from build123d import *

# Parameters (mm, degrees)
SKETCH_2_R               = 4
SKETCH_2_R_2             = 2
SKETCH_2_R_3             = 2.5
SKETCH_2_R_4             = 1.5
SKETCH_2_R_5             = 2.125
SKETCH_2_R_6             = 1
EXTRUDE_1_DEPTH          = 17.125
CUT_EXTRUDE_1_DEPTH      = 137.144257132
CUT_EXTRUDE_1_DEPTH_BACK = 137.144257132
SKETCH_3_W               = 6.985996156
SKETCH_3_H               = 14.275
CUT_EXTRUDE_START        = -128.325
CUT_EXTRUDE_2_OUTLINE_W  = 32
CUT_EXTRUDE_2_OUTLINE_H  = 0.125
CUT_EXTRUDE_2_DEPTH      = 16.325


# Read off the part's stored shape, not the designer's step: 切除-拉伸2
with BuildPart() as part:
    # 草图2 → 凸台-拉伸1 (new body)
    # profile 1 of 4: a face of its own
    with BuildSketch(Plane.XY.offset(8.375)):
        with BuildLine():
            Line((-15.5, -121), (-15.5, -116))
            Line((-15.5, -116), (-17.125, -116))
            ThreePointArc((-17.125, -116), (-23.953427125, -118.828427125), (-21.125, -112))
            Line((-21.125, -112), (-35.875, -112))
            ThreePointArc((-35.875, -112), (-34.107233047, -112.732233047), (-33.375, -114.5))
            ThreePointArc((-33.375, -114.5), (-35.875, -117), (-38.375, -114.5))
            Line((-38.375, -114.5), (-38.375, -118.75))
            Line((-38.375, -118.75), (-43.26696162, -120.643234405))
            ThreePointArc((-43.26696162, -120.643234405), (-41.298785706, -120.872085507), (-40.375, -122.625))
            ThreePointArc((-40.375, -122.625), (-41.477365663, -124.487751731), (-43.640735541, -124.417860124))
            Line((-43.640735541, -124.417860124), (-37.5, -128.325))
            Line((-37.5, -128.325), (-23, -128.325))
            Line((-23, -128.325), (-15.5, -121))
        make_face()
    # profile 2 of 4: a face of its own
    with BuildSketch(Plane.XY.offset(8.375)):
        with Locations((-21.125, -116)):
            Circle(SKETCH_2_R)
        with Locations((-21.125, -116)):
            Circle(SKETCH_2_R_2, mode=Mode.SUBTRACT)
    # profile 3 of 4: a face of its own
    with BuildSketch(Plane.XY.offset(8.375)):
        with Locations((-35.875, -114.5)):
            Circle(SKETCH_2_R_3)
        with Locations((-35.875, -114.5)):
            Circle(SKETCH_2_R_4, mode=Mode.SUBTRACT)
    # profile 4 of 4: a face of its own
    with BuildSketch(Plane.XY.offset(8.375)):
        with Locations((-42.5, -122.625)):
            Circle(SKETCH_2_R_5)
        with Locations((-42.5, -122.625)):
            Circle(SKETCH_2_R_6, mode=Mode.SUBTRACT)
    extrude(amount=-EXTRUDE_1_DEPTH)

    # 草图3 → 切除-拉伸1 (cut, two sides: drawn at the far end of the back side and taken through both)
    with BuildSketch(Plane(origin=(0, 0, 0), x_dir=(1, 0, 0), z_dir=(0, 1, 0)).offset(-CUT_EXTRUDE_1_DEPTH_BACK)):
        with Locations((-42.942998078, 0.1875)):
            Rectangle(SKETCH_3_W, SKETCH_3_H)
    extrude(amount=CUT_EXTRUDE_1_DEPTH + CUT_EXTRUDE_1_DEPTH_BACK, mode=Mode.SUBTRACT)

    # 切除-拉伸2 outline → 切除-拉伸2 (cut)
    with BuildSketch(Plane(origin=(0, 0, 0), x_dir=(1, 0, 0), z_dir=(0, 1, 0)).offset(CUT_EXTRUDE_START)):
        with Locations((-30, -8.3125)):
            Rectangle(CUT_EXTRUDE_2_OUTLINE_W, CUT_EXTRUDE_2_OUTLINE_H)
        with Locations((-30, 8.6875)):
            Rectangle(CUT_EXTRUDE_2_OUTLINE_W, CUT_EXTRUDE_2_OUTLINE_H)
    extrude(amount=CUT_EXTRUDE_2_DEPTH, mode=Mode.SUBTRACT)


solid = part.part
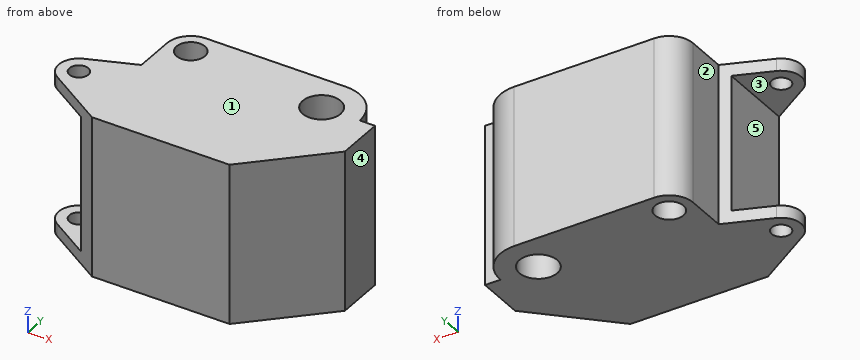
For this review, take the finished solid that the model builds, in its own axes (mm). Face numbers are marked on the shaded views. A direction names the side the tool comes from. Round coordinates to 2 decimals unless told otherwise and drop trailing zeros. Loops run counter-clockwise (first coordinate to the right, second up) from the corner with the lowest first, then second, coordinate; pieces in that order, holes last. Notation, with made-up numbers: (-28.5, 58.25) - (-24.5, 58.25) arc R13 ccw to (-24.5, 70.25) - close; hole circle Ø10 at (68, -36.5). An arc over 180 degrees is marked (long way). Answer as CSV lines item,"result".
(1) Insertion check: P1, Ø1, axis at x = -19.5, z = -0.5, coming from the +Y side; P2, Ø0.5, axis at x = -16.5, z = -0.5, coming from the +Y side; P3, Ø4, axis at y = -121.5, z = -1, coming from the -X side. Each pin has a flat end and moves straight along its axis. Give the tip position at first contact, or say it passes through.
Checked values:
P1,"stops at y = -112.16"
P2,"stops at y = -116"
P3,"stops at x = -39.45"
(2) Wall thickness on line 1 (Z direction, x = -41.25, y = -120.5) (3 decimals); line 2 (X direction, y = -114.5, z = -5) (3 decimals); line 3 (Y direction, x = -42.75, z = 7.5): over which ranges is each line inside the solid? List them lowest first.
Checked values:
line 1,"z = -8.625 to -7.325, 6.95 to 8.25"
line 2,"x = -38.375 to -37.375, -34.375 to -22.448, -19.802 to -17.417"
line 3,"y = -124.98 to -123.59, -121.66 to -120.44"
(3) Consider section B-B on x = -40. Give the boundary of the cut face in (y, z) (3 decimals).
Checked values:
outline,"(-126.734, -8.625) - (-119.379, -8.625) - (-119.379, -7.325) - (-126.734, -7.325) - close; (-126.734, 6.95) - (-119.379, 6.95) - (-119.379, 8.25) - (-126.734, 8.25) - close"
(4) Tool access review of the marked faces 4 and 5: name each direction out of +Z, -Z, +X, -X, +Y, -Y from which nothing blocks a thin tool from reaching the whole face with its end or side.
Checked values:
face 4,"+Z, -Z, +X, +Y, -Y"
face 5,"-X, +Y, -Y"
(5) Consider section C-C on y = -117. Give the boundary of the cut face in (x, z) (3 decimals), then the cut area to 3 significant figures.
Checked values:
outline,"(-38.375, -8.625) - (-22.857, -8.625) - (-22.857, 8.25) - (-38.375, 8.25) - close; (-19.393, -8.625) - (-15.5, -8.625) - (-15.5, 8.25) - (-19.393, 8.25) - close"
area,"328 mm2"
(6) Mouldability with a two-part tool opening along Z and no side actions: class the marked faces 1, 2 and 3 as +Z half, -Z half, draft (parallel to the pull), parting line (faces both ways), or undercut.
Checked values:
face 1,"+Z half"
face 2,"draft"
face 3,"undercut"
(7) Consider section A-A on z = -5. Give the boundary of the cut face in (x, y) (3 decimals).
Checked values:
outline,"(-39.45, -127.084) - (-37.5, -128.325) - (-23, -128.325) - (-15.5, -121) - (-15.5, -116) - (-17.125, -116) arc R4 ccw to (-21.125, -112) - (-35.875, -112) arc R2.5 ccw to (-38.375, -114.5) - (-38.375, -118.75) - (-39.45, -119.166) - close; hole circle Ø3 at (-35.875, -114.5); hole circle Ø4 at (-21.125, -116)"
